```python
from build123d import *

# Parameters (mm, degrees)
SKICA1_W                = 7.14
SKICA1_H                = 2.36
P_IDAT_VYSUNUT_M1_DEPTH = 2.5
SKICA2_W                = 0.58
SKICA2_H                = 0.58
P_IDAT_VYSUNUT_M2_DEPTH = 5.9
LINPOLE1_COUNT          = 3
LINPOLE1_PITCH          = 2.44


with BuildPart() as part:
    # Skica1 → Přidat vysunutím1 (new body)
    with BuildSketch(Plane.XY):
        Rectangle(SKICA1_W, SKICA1_H)
    extrude(amount=P_IDAT_VYSUNUT_M1_DEPTH)

    # Skica2 → Přidat vysunutím2 (add)
    with BuildSketch(Plane.XY.offset(2.5)):
        with Locations((2.44, 0)):
            Rectangle(SKICA2_W, SKICA2_H)
    p_idat_vysunut_m2 = extrude(amount=P_IDAT_VYSUNUT_M2_DEPTH)

    # LinPole1: Přidat vysunutím2 ×3
    with Locations(*[(-i * LINPOLE1_PITCH, 0, 0) for i in range(1, LINPOLE1_COUNT)]):
        add(p_idat_vysunut_m2)


solid = part.part
```
Model file for the job. Use its own axes, mm. Round coordinates to 2 decimals unless told otherwise and drop trailing zeros. Write each loop counter-clockwise with the first axis right and the second up, starting at its lowest first coordinate (ties: lowest second). Pieces come first, ordered by that corner, then holes. Notation, with made-up numbers: M 44.25,36 L 94.25,36 A6 cw 94.25,44 Z; hole C 41,-24.75 d7. An arc over 180 degrees is marked long. Put each result on its own line as item: value.
Item 1: Flat gauge pins, fed straight in: P1, Ø0.6, axis at x = 2.5, z = 6, coming from the +Y side; P2, Ø0.6, axis at y = 0, z = 6, coming from the -X side; P3, Ø0.6, axis at x = 2.5, z = 5.5, coming from the -Y side. Where does each tip first touch, or does it go through?
Responses:
P1: y = 0.29
P2: x = -2.73
P3: y = -0.29
Item 2: Cut at B-B (x = -2.5). List the corners of the cut face in (y, z), and give its area (3 significant figures).
Responses:
outline: M -1.18,0 L 1.18,0 L 1.18,2.5 L 0.29,2.5 L 0.29,8.4 L -0.29,8.4 L -0.29,2.5 L -1.18,2.5 Z
area: 9.32 mm²
Item 3: Cut at A-A (z = 6.75). List the corners of the cut face in (x, y).
Responses:
outline: M -2.73,-0.29 L -2.15,-0.29 L -2.15,0.29 L -2.73,0.29 Z; M -0.29,-0.29 L 0.29,-0.29 L 0.29,0.29 L -0.29,0.29 Z; M 2.15,-0.29 L 2.73,-0.29 L 2.73,0.29 L 2.15,0.29 Z
Item 4: Cut at D-D (x = 1). List the corners of the cut face in (y, z).
Responses:
outline: M -1.18,0 L 1.18,0 L 1.18,2.5 L -1.18,2.5 Z
Item 5: Cut at C-C (y = -0.05). List the corners of the cut face in (x, z), and give its area (3 significant figures).
Responses:
outline: M -3.57,0 L 3.57,0 L 3.57,2.5 L 2.73,2.5 L 2.73,8.4 L 2.15,8.4 L 2.15,2.5 L 0.29,2.5 L 0.29,8.4 L -0.29,8.4 L -0.29,2.5 L -2.15,2.5 L -2.15,8.4 L -2.73,8.4 L -2.73,2.5 L -3.57,2.5 Z
area: 28.1 mm²
Item 6: Probe L1, parallel to X at y = -0.25, z = 3.25; L2, parallel to Z at x = 3, y = 0.8. List the from-to ranges inside material, lowest first. Write a range as from..to.
Responses:
L1: -2.73..-2.15, -0.29..0.29, 2.15..2.73
L2: 0..2.5
